from build123d import *

# Parameters (mm, degrees)
F3_R     = 6
F4_DEPTH = 25


with BuildPart() as f1:
    # F0 (on Front) → F1 (revolve)
    with BuildSketch(Plane.XZ):
        Polygon((-80.545663, 183.5), (-80.545663, 124), (-77.545663, 124), (-77.545663, 114.5), (-15.382721, 102.5), (108.119988, 143.666695), (108.119988, 162.5), (112.119988, 162.5), (112.119988, 165), (-37.880012, 165), (-52.880012, 165), (-66.545663, 183.5), align=None)
    revolve(axis=Axis((211.105403, 0, 82.5), (1, 0, 0)))

    # F3 (on face) → F4 (cut)
    with BuildSketch(Plane.YZ.offset(108.119988)):
        with Locations((-22.803705, 147.569913)):
            Circle(F3_R)
        with Locations((-67.75405, 95.286369)):
            Circle(F3_R)
        with Locations((-44.950345, 30.216456)):
            Circle(F3_R)
        with BuildLine():
            ThreePointArc((17.060371, 15.693966), (23.681201, 11.494601), (28.803705, 17.430087))
            ThreePointArc((28.803705, 17.430087), (21.926209, 23.365574), (17.060371, 15.693966))
        make_face()
        with Locations((67.75405, 69.713631)):
            Circle(F3_R)
        with Locations((44.950345, 134.783544)):
            Circle(F3_R)
    extrude(amount=-F4_DEPTH, mode=Mode.SUBTRACT)


solid = f1.part
Verification items for the finished model (mm, model axes). A direction names the side the tool comes from. Give positions to 0.01 mm unless a question says otherwise; leave off trailing zeros. Write each loop counter-clockwise with the first axis right and the second up, starting at its lowest first coordinate (ties: lowest second). Pieces come first, ordered by that corner, then holes. Notation, with made-up numbers: (28, 85) - (83, 85) arc R13 cw to (83, 108) - close; hole circle Ø2 at (73, 36.5). An arc over 180 degrees is marked (long way). Answer as CSV lines item,"result". Start each with the question number.
1. Sectioned sample at C-C (x = 55). Record the boundary of the cut face in (y, z).
2. Sectioned sample at A-A (z = 82.5). Record the boundary of the cut face in (x, y), then the cut area to 3 significant figures.
3. Draft check along Y on faces 4 (the face through (28.46, 50.2, 17.03)), 5 (the face through (83.12, 23, 18)), 6 (the face through (-80.546, 43, 81)). Enter one of: pulls with the +Y half, pulls with the -Y half, needs draft (parallel to the pull), parting line crosses it, or undercut.
4. Depth check by flat-ended pin: pin 1 (13 mm diameter, centred on y = -23, z = 147.5, fed in from +X); pin 2 (8 mm diameter, centred on x = 5, z = 44, fed in from +Y); pin 3 (10 mm diameter, centred on x = 91, z = 70.5, fed in from +Y). Enter the tip coordinate at first touch or a pass-through.
5. Set-up check for faces 1 (the face through (112.12, -43.2, 150.1)), 2 (the face through (95.79, -62.21, 92.99)), 3 (the face through (-79.025, -12.465, 122.084)): record each of +Z, -Z, +X, -X, +Y, -Y from which the full face is reachable in a straight line by a thin tool's end or side.
6. Sectioned sample at D-D (x = -58). Record the boundary of the cut face in (y, z).
7. Thickness scan on line 1 (Z direction, x = -78.85, y = 0); line 2 (Z direction, x = 57.5, y = -17.5); line 3 (Y direction, x = 43, z = 65). Record the ranges inside material, lowest first.
8. Sectioned sample at B-B (y = 0). Record the boundary of the cut face in (x, z), then the cut area to 3 significant figures.
Derived:
1,outline,"circle Ø165 at (0, 82.5); hole circle Ø86.92 at (0, 82.5)"
2,outline,"(-80.55, -101) - (-66.55, -101) - (-52.88, -82.5) - (112.12, -82.5) - (112.12, -80) - (108.12, -80) - (108.12, -61.17) - (-15.38, -20) - (-77.55, -32) - (-77.55, -41.5) - (-80.55, -41.5) - close; (-80.55, 41.5) - (-77.55, 41.5) - (-77.55, 32) - (-15.38, 20) - (108.12, 61.17) - (108.12, 80) - (112.12, 80) - (112.12, 82.5) - (-52.88, 82.5) - (-66.55, 101) - (-80.55, 101) - close"
2,area,"18,400 mm²"
3,face 4,"parting line crosses it"
3,face 5,"undercut"
3,face 6,"needs draft"
4,pin 1,"x = 108.12"
4,pin 2,"y = 74.94"
4,pin 3,"y = 82.2"
5,face 1,"+Z, -Z, +X, +Y, -Y"
5,face 2,"+X"
5,face 3,"-X"
6,outline,"circle Ø178.86 at (0, 82.5); hole circle Ø56.45 at (0, 82.5)"
7,line 1,"-18.5 to 41, 124 to 183.5"
7,line 2,"1.88 to 41.81, 123.19 to 163.12"
7,line 3,"-80.62 to -35.37, 35.37 to 80.62"
8,outline,"(-80.55, -18.5) - (-66.55, -18.5) - (-52.88, 0) - (112.12, 0) - (112.12, 2.5) - (108.12, 2.5) - (108.12, 21.33) - (-15.38, 62.5) - (-77.55, 50.5) - (-77.55, 41) - (-80.55, 41) - close; (-80.55, 124) - (-77.55, 124) - (-77.55, 114.5) - (-15.38, 102.5) - (108.12, 143.67) - (108.12, 162.5) - (112.12, 162.5) - (112.12, 165) - (-52.88, 165) - (-66.55, 183.5) - (-80.55, 183.5) - close"
8,area,"18,400 mm²"
